Geometry check sheet. Reference: the model listing, model coordinates, mm. Coordinates: 2 decimals unless noted, no trailing zeros. Write each loop counter-clockwise with the first axis right and the second up, starting at its lowest first coordinate (ties: lowest second). Pieces come first, ordered by that corner, then holes.
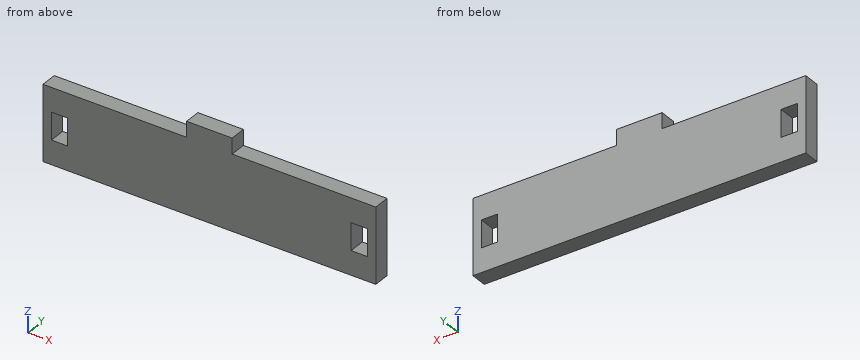
from build123d import *

# Parameters (mm, degrees)
F0_W     = 3.175
F0_H     = 5.334
F1_DEPTH = 3.175


with BuildPart() as f1:
    # F0 (on Front) → F1 (new body)
    with BuildSketch(Plane.XZ):
        Polygon((-32.512, 7.366), (-32.512, -7.366), (-12.827, -7.366), (18.288, -7.366), (32.512, -7.366), (32.512, 7.366), (4.445, 7.366), (4.445, 10.414), (-4.445, 10.414), (-4.445, 7.366), align=None)
        with Locations((-29.2735, 0)):
            Rectangle(F0_W, F0_H, mode=Mode.SUBTRACT)
        with Locations((29.2735, 0)):
            Rectangle(F0_W, F0_H, mode=Mode.SUBTRACT)
    extrude(amount=F1_DEPTH)


solid = f1.part
1. Thickness scan on line 1 along X through (y, z) = (-0.35, -0.25); line 2 along Z through (x, y) = (16, -1.4); line 3 along X through (y, z) = (-0.45, 7.5) (3 decimals). Record the ranges inside material, lowest first.
Computed values:
line 1: x = -32.51 to -30.86, -27.69 to 27.69, 30.86 to 32.51
line 2: z = -7.37 to 7.37
line 3: x = -4.445 to 4.445
2. Gauge pin test, flat end, axial feed: pin 1 Ø1.6 at (x, y) = (-29.5, -2) entering from +Z. Record the tip position at first contact, or that the pin passes through.
Computed values:
pin 1: stops at z = 7.37
3. Sectioned sample at C-C, the plane x = -6.5. Record the boundary of the cut face in (y, z) (3 decimals), and give its area (3 significant figures).
Computed values:
outline: (-3.175, -7.366) - (0, -7.366) - (0, 7.366) - (-3.175, 7.366) - close
area: 46.8 mm2
4. Sectioned sample at A-A, the plane y = -2.45. Record the boundary of the cut face in (x, z) (3 decimals).
Computed values:
outline: (-32.512, -7.366) - (32.512, -7.366) - (32.512, 7.366) - (4.445, 7.366) - (4.445, 10.414) - (-4.445, 10.414) - (-4.445, 7.366) - (-32.512, 7.366) - close; hole (-30.861, -2.667) - (-27.686, -2.667) - (-27.686, 2.667) - (-30.861, 2.667) - close; hole (27.686, -2.667) - (30.861, -2.667) - (30.861, 2.667) - (27.686, 2.667) - close
5. Sectioned sample at B-B, the plane z = 0.5. Record the boundary of the cut face in (x, y) (3 decimals).
Computed values:
outline: (-32.512, -3.175) - (-30.861, -3.175) - (-30.861, 0) - (-32.512, 0) - close; (-27.686, -3.175) - (27.686, -3.175) - (27.686, 0) - (-27.686, 0) - close; (30.861, -3.175) - (32.512, -3.175) - (32.512, 0) - (30.861, 0) - close
